```python
from build123d import *

# Parameters (mm, degrees)
SKETCH1_W           = 20
SKETCH1_H           = 4
SKETCH1_W_2         = 4
SKETCH1_H_2         = 20
BOSS_EXTRUDE1_DEPTH = 4
CUT_EXTRUDE1_DEPTH  = 10
SKETCH3_R           = 4
CUT_EXTRUDE2_DEPTH  = 10


with BuildPart() as part:
    # Sketch1 → Boss-Extrude1 (new body)
    with BuildSketch(Plane(origin=(0, 0, 0), x_dir=(0, 0, -1), z_dir=(1, 0, 0))):
        Polygon((-401.564712347, -166), (-381.564712347, -166), (-381.564712347, -170), (-361.564712347, -170), (-361.564712347, -166), (-244.564712347, -166), (-244.564712347, -170), (-224.564712347, -170), (-224.564712347, -166), (-107.564712347, -166), (-107.564712347, -170), (-87.564712347, -170), (-87.564712347, -166), (29.435287653, -166), (29.435287653, -170), (49.435287653, -170), (49.435287653, -166), (166.435287653, -166), (166.435287653, -170), (186.435287653, -170), (186.435287653, -166), (208.435287653, -166), (208.435287653, 236), (186.435287653, 236), (186.435287653, 240), (166.435287653, 240), (166.435287653, 236), (49.435287653, 236), (49.435287653, 240), (29.435287653, 240), (29.435287653, 236), (-87.564712347, 236), (-87.564712347, 240), (-107.564712347, 240), (-107.564712347, 236), (-224.564712347, 236), (-224.564712347, 240), (-244.564712347, 240), (-244.564712347, 236), (-361.564712347, 236), (-361.564712347, 240), (-381.564712347, 240), (-381.564712347, 236), (-401.564712347, 236), align=None)
        with Locations((190.435287653, -57)):
            Rectangle(SKETCH1_W, SKETCH1_H, mode=Mode.SUBTRACT)
        with Locations((38.825287653, 32)):
            Rectangle(SKETCH1_W_2, SKETCH1_H_2, mode=Mode.SUBTRACT)
        with Locations((38.825287653, -146)):
            Rectangle(SKETCH1_W_2, SKETCH1_H_2, mode=Mode.SUBTRACT)
        with Locations((-395.564712347, 216)):
            Rectangle(SKETCH1_W_2, SKETCH1_H_2, mode=Mode.SUBTRACT)
        with Locations((-395.564712347, 106)):
            Rectangle(SKETCH1_W_2, SKETCH1_H_2, mode=Mode.SUBTRACT)
        with Locations((-395.564712347, -36)):
            Rectangle(SKETCH1_W_2, SKETCH1_H_2, mode=Mode.SUBTRACT)
        with Locations((-395.564712347, -146)):
            Rectangle(SKETCH1_W_2, SKETCH1_H_2, mode=Mode.SUBTRACT)
        with Locations((202.435287653, 216)):
            Rectangle(SKETCH1_W_2, SKETCH1_H_2, mode=Mode.SUBTRACT)
        with Locations((202.435287653, 106)):
            Rectangle(SKETCH1_W_2, SKETCH1_H_2, mode=Mode.SUBTRACT)
        with Locations((202.435287653, -36)):
            Rectangle(SKETCH1_W_2, SKETCH1_H_2, mode=Mode.SUBTRACT)
        with Locations((202.435287653, -146)):
            Rectangle(SKETCH1_W_2, SKETCH1_H_2, mode=Mode.SUBTRACT)
        with Locations((190.435287653, 54)):
            Rectangle(SKETCH1_W, SKETCH1_H, mode=Mode.SUBTRACT)
        with Locations((-231.954712347, -146)):
            Rectangle(SKETCH1_W_2, SKETCH1_H_2, mode=Mode.SUBTRACT)
        with Locations((-231.954712347, 32)):
            Rectangle(SKETCH1_W_2, SKETCH1_H_2, mode=Mode.SUBTRACT)
        with Locations((-383.564712347, 54)):
            Rectangle(SKETCH1_W, SKETCH1_H, mode=Mode.SUBTRACT)
        with Locations((-278.564712347, 54)):
            Rectangle(SKETCH1_W, SKETCH1_H, mode=Mode.SUBTRACT)
        with Locations((-173.564712347, 54)):
            Rectangle(SKETCH1_W, SKETCH1_H, mode=Mode.SUBTRACT)
        with Locations((85.435287653, 54)):
            Rectangle(SKETCH1_W, SKETCH1_H, mode=Mode.SUBTRACT)
        with Locations((-19.564712347, 54)):
            Rectangle(SKETCH1_W, SKETCH1_H, mode=Mode.SUBTRACT)
        with Locations((-248.564712347, -57)):
            Rectangle(SKETCH1_W, SKETCH1_H, mode=Mode.SUBTRACT)
        with Locations((-383.564712347, -57)):
            Rectangle(SKETCH1_W, SKETCH1_H, mode=Mode.SUBTRACT)
        with Locations((55.435287653, -57)):
            Rectangle(SKETCH1_W, SKETCH1_H, mode=Mode.SUBTRACT)
    extrude(amount=BOSS_EXTRUDE1_DEPTH)

    # Sketch2 → Cut-Extrude1 (cut)
    with BuildSketch(Plane(origin=(4, 0, 0), x_dir=(0, 0, -1), z_dir=(1, 0, 0))):
        with BuildLine():
            Line((-170.064712347, 9), (-25.064712347, 9))
            ThreePointArc((-25.064712347, 9), (-7.387042818, 1.67766953), (-0.064712347, -16))
            Line((-0.064712347, -16), (-0.064712347, -106))
            ThreePointArc((-0.064712347, -106), (-7.387042818, -123.67766953), (-25.064712347, -131))
            Line((-25.064712347, -131), (-170.064712347, -131))
            ThreePointArc((-170.064712347, -131), (-187.742381877, -123.67766953), (-195.064712347, -106))
            Line((-195.064712347, -106), (-195.064712347, -16))
            ThreePointArc((-195.064712347, -16), (-187.742381877, 1.67766953), (-170.064712347, 9))
        make_face()
        with BuildLine():
            Line((-169.064712347, 201), (-24.064712347, 201))
            ThreePointArc((-24.064712347, 201), (-6.387042818, 193.67766953), (0.935287653, 176))
            Line((0.935287653, 176), (0.935287653, 86))
            ThreePointArc((0.935287653, 86), (-6.387042818, 68.32233047), (-24.064712347, 61))
            Line((-24.064712347, 61), (-169.064712347, 61))
            ThreePointArc((-169.064712347, 61), (-186.742381877, 68.32233047), (-194.064712347, 86))
            Line((-194.064712347, 86), (-194.064712347, 176))
            ThreePointArc((-194.064712347, 176), (-186.742381877, 193.67766953), (-169.064712347, 201))
        make_face()
        with BuildLine():
            Line((-336.564712347, 178.5), (-281.564712347, 178.5))
            ThreePointArc((-281.564712347, 178.5), (-263.887042818, 171.17766953), (-256.564712347, 153.5))
            Line((-256.564712347, 153.5), (-256.564712347, 108.5))
            ThreePointArc((-256.564712347, 108.5), (-263.887042818, 90.82233047), (-281.564712347, 83.5))
            Line((-281.564712347, 83.5), (-336.564712347, 83.5))
            ThreePointArc((-336.564712347, 83.5), (-354.242381877, 90.82233047), (-361.564712347, 108.5))
            Line((-361.564712347, 108.5), (-361.564712347, 153.5))
            ThreePointArc((-361.564712347, 153.5), (-354.242381877, 171.17766953), (-336.564712347, 178.5))
        make_face()
        with BuildLine():
            Line((88.435287653, 178.5), (143.435287653, 178.5))
            ThreePointArc((143.435287653, 178.5), (161.112957182, 171.17766953), (168.435287653, 153.5))
            Line((168.435287653, 153.5), (168.435287653, 108.5))
            ThreePointArc((168.435287653, 108.5), (161.112957182, 90.82233047), (143.435287653, 83.5))
            Line((143.435287653, 83.5), (88.435287653, 83.5))
            ThreePointArc((88.435287653, 83.5), (70.757618123, 90.82233047), (63.435287653, 108.5))
            Line((63.435287653, 108.5), (63.435287653, 153.5))
            ThreePointArc((63.435287653, 153.5), (70.757618123, 171.17766953), (88.435287653, 178.5))
        make_face()
    extrude(amount=-CUT_EXTRUDE1_DEPTH, mode=Mode.SUBTRACT)

    # Sketch3 → Cut-Extrude2 (cut)
    with BuildSketch(Plane(origin=(4, 0, 0), x_dir=(0, 0, -1), z_dir=(1, 0, 0))):
        with Locations((-382.564712347, 136.477800328)):
            Circle(SKETCH3_R)
        with Locations((189.435287653, 136.477800328)):
            Circle(SKETCH3_R)
    extrude(amount=-CUT_EXTRUDE2_DEPTH, mode=Mode.SUBTRACT)


solid = part.part
```
Geometry check sheet. Reference: the model listing, model coordinates, mm. A direction names the side the tool comes from. Coordinates: 2 decimals unless noted, no trailing zeros. Order: outer loops, then holes, each group sorted by start corner. A loop starts at its lowest first (then second) coordinate and runs counter-clockwise, first axis right, second up. Notation, with made-up numbers: M 59,-19.5 L 95,-19.5 A10 ccw 95,-14.5 Z; hole C 84.25,25 d6. An arc over 180 degrees is marked long. One line per question, with ' | ' between items. Start each with the question number.
Item 1: Set-up check for faces 3 (the flat face through (0, 38, 101)), 4 (the cylindrical face through (2.03, 170.98, 354.44)): record each of +Z, -Z, +X, -X, +Y, -Y from which the full face is reachable in a straight line by a thin tool's end or side.
Item 2: Gauge pin test, flat ends, axial feed: pin 1 (1.2 mm diameter, centred on x = 2.5, z = 173, fed in from +Y); pin 2 (1.2 mm diameter, centred on x = 1, y = -169, fed in from -Z); pin 3 (2 mm diameter, centred on x = 3, z = 395.5, fed in from -Y). Record the tip position at first contact, or that the pin passes through.
Item 3: Cross-section at D-D on x = 2.25. State how many separate pieces and enclosed holes the cut face has, then the cut area to 3 significant figures.
Item 4: Cross-section at A-A on z = 150.5. Enter the section's corners in (x, y), then the cut area to 3 significant figures.
Item 5: Draft check along Y on faces 1 (the flat face through (4, 38, 101)), 2 (the cylindrical face through (2.03, 193.87, 6.58)). Enter one of: pulls with the +Y half, pulls with the -Y half, needs draft (parallel to the pull), parting line crosses it, or undercut.
Item 6: Cross-section at C-C on z = 319.5. Enter the section's corners in (x, y).
Item 7: Material ranges on L1, parallel to Y at x = 2.6, z = 161; L2, parallel to Z at x = 0.9, y = 208.5; L3, parallel to Z at x = 2.45, y = -101.5, recorded low to high. Write a range as [from, to].
Item 8: Cross-section at B-B on y = -88. Enter the section's corners in (x, z).
Findings:
1) face 3: +Z, -Z, -X, +Y, -Y | face 4: +X, -X
2) pin 1: stops at y = 236 | pin 2: stops at z = -186.44 | pin 3: stops at y = -166
3) separate pieces: 1 | enclosed holes: 28 | area: 172,000 mm²
4) outline: M 0,-166 L 4,-166 L 4,-131 L 0,-131 Z; M 0,9 L 4,9 L 4,61 L 0,61 Z; M 0,201 L 4,201 L 4,236 L 0,236 Z | area: 488 mm²
5) face 1: needs draft | face 2: undercut
6) outline: M 0,-166 L 4,-166 L 4,83.5 L 0,83.5 Z; M 0,178.5 L 4,178.5 L 4,236 L 0,236 Z
7) L1: y = [-166, -131], [9, 61], [201, 236] | L2: z = [-208.44, -204.44], [-200.44, 393.56], [397.56, 401.56] | L3: z = [-208.44, 0.06], [195.06, 401.56]
8) outline: M 0,-208.44 L 4,-208.44 L 4,0.06 L 0,0.06 Z; M 0,195.06 L 4,195.06 L 4,401.56 L 0,401.56 Z
